Geometry: see drawing. Coordinates: mm, zero at the bounding-box minimum. A direction names the side the tool comes from. Give positions to 0.01 mm unless a question says otherwise; leave off trailing zeros. Loops run counter-clockwise (first coordinate to the right, second up) from the corner with the lowest first, then second, coordinate; pieces in that order, holes last. Notation, with made-up numbers: (-19.75, -38) -> (-11.75, -38) arc R20 ccw to (-11.75, -29) -> close; hole circle Ø4 at (58.25, 73). An arc over 180 degrees is marked (long way). Use CSV: the item, a comma, the result in double quotes.
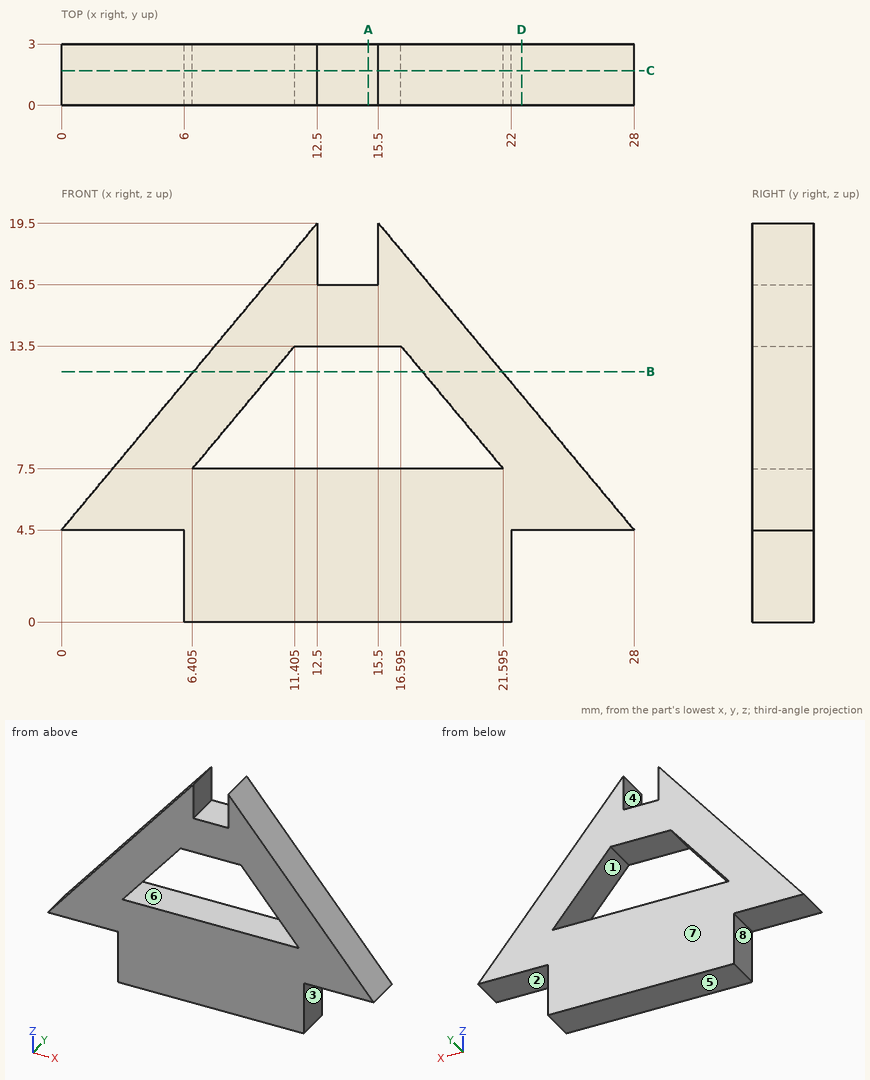
1) Section query C-C (y = 1.7). Return loops of the section in (x, z) (3 decimals).
From the geometry:
outline,"(0, 4.5) -> (6, 4.5) -> (6, 0) -> (22, 0) -> (22, 4.5) -> (28, 4.5) -> (15.5, 19.5) -> (15.5, 16.5) -> (12.5, 16.5) -> (12.5, 19.5) -> close; hole (6.405, 7.5) -> (21.595, 7.5) -> (16.595, 13.5) -> (11.405, 13.5) -> close"
2) Reachability of the marked faces 4, 5, 6, 7 and 8 from +Z, -Z, +X, -X, +Y, -Y: full face, straight path, thin tool, end or side. Return the list, or none.
From the geometry:
face 4,"+Z, +Y, -Y"
face 5,"-Z, +X, -X, +Y, -Y"
face 6,"+Y, -Y"
face 7,"+Z, -Z, +X, -X, +Y"
face 8,"-Z, -X, +Y, -Y"
3) Section query D-D (x = 22.5). Return loops of the section in (y, z).
From the geometry:
outline,"(0, 4.5) -> (3, 4.5) -> (3, 11.1) -> (0, 11.1) -> close"
4) Section query A-A (x = 15). Return loops of the section in (y, z), then the cut area to 3 significant figures.
From the geometry:
outline,"(0, 0) -> (3, 0) -> (3, 7.5) -> (0, 7.5) -> close; (0, 13.5) -> (3, 13.5) -> (3, 16.5) -> (0, 16.5) -> close"
area,"31.5 mm^2"
5) Ray query, line 1 (Z direction, x = 15.25, y = 2.5); line 2 (X direction, y = 1.85, z = 2.25); line 3 (Z direction, x = 10, y = 2.45). Return the intervals inside material, ascending.
From the geometry:
line 1,"z = 0 to 7.5, 13.5 to 16.5"
line 2,"x = 6 to 22"
line 3,"z = 0 to 7.5, 11.81 to 16.5"
6) Contact query for flat-ended pins moving along their axis: pin 1 (1.5 mm diameter, centred on x = 13.5, y = 1.5, fed in from +Z); pin 2 (1.5 mm diameter, centred on y = 2, z = 2.5, fed in from +X); pin 3 (1.5 mm diameter, centred on y = 2, z = 1.5, fed in from -X). Output: stop coordinate, or through.
From the geometry:
pin 1,"stops at z = 16.5"
pin 2,"stops at x = 22"
pin 3,"stops at x = 6"
7) Section query B-B (z = 12.25). Return loops of the section in (x, y).
From the geometry:
outline,"(6.46, 0) -> (10.36, 0) -> (10.36, 3) -> (6.46, 3) -> close; (17.64, 0) -> (21.54, 0) -> (21.54, 3) -> (17.64, 3) -> close"
8) Mould query, pull axis X, two halves, no side actions, for the marked faces 1, 2 and 3. Classes: pulls with the +X half, pulls with the -X half, needs draft (parallel to the pull), parting line crosses it, or undercut.
From the geometry:
face 1,"undercut"
face 2,"needs draft"
face 3,"pulls with the +X half"
